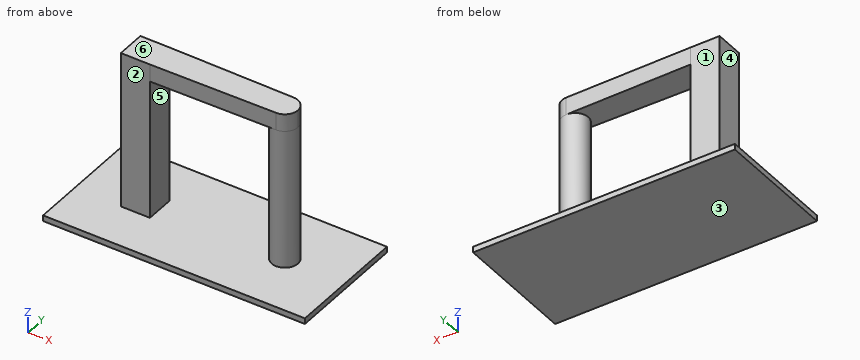
from build123d import *

# Parameters (mm, degrees)
F0_W     = 45
F0_H     = 21
F0_W_2   = 5
F0_H_2   = 5
F0_R     = 2.25
F1_DEPTH = 1
F2_DEPTH = 25
F3_W     = 5
F3_H     = 5
F4_DEPTH = 3


with BuildPart() as f1:
    # F0 (on Top) → F1 (new body)
    with BuildSketch(Plane.XY):
        Rectangle(F0_W, F0_H)
        with Locations((-12, 0)):
            Rectangle(F0_W_2, F0_H_2, mode=Mode.SUBTRACT)
        with Locations((12, 0)):
            Circle(F0_R, mode=Mode.SUBTRACT)
    extrude(amount=F1_DEPTH)

    # F0 (on Top) → F2 (join)
    with BuildSketch(Plane.XY):
        with Locations((-12, 0)):
            Rectangle(F0_W_2, F0_H_2)
        with Locations((12, 0)):
            Circle(F0_R)
    extrude(amount=F2_DEPTH)

    # F3 (on face) → F4 (join)
    with BuildSketch(Plane.XY.offset(25)):
        with BuildLine():
            Line((12.026145, 2.249848), (-9.5, 2.5))
            Line((-9.5, 2.5), (-9.5, -2.5))
            Line((-9.5, -2.5), (12.026145, -2.249848))
            ThreePointArc((12.026145, -2.249848), (9.75, 0), (12.026145, 2.249848))
        make_face()
        with Locations((-12, 0)):
            Rectangle(F3_W, F3_H)
        with BuildLine():
            ThreePointArc((14.25, 0), (13.600207, 1.58172), (12.026145, 2.249848))
            ThreePointArc((12.026145, 2.249848), (9.75, 0), (12.026145, -2.249848))
            ThreePointArc((12.026145, -2.249848), (13.600207, -1.58172), (14.25, 0))
        make_face()
    extrude(amount=F4_DEPTH)


solid = f1.part
The listing builds one solid part. Answer for the finished solid, in the listing's coordinates (mm). Face numbers are marked on the shaded views. A direction names the side the tool comes from. Give positions to 0.01 mm unless a question says otherwise; leave off trailing zeros. Write each loop counter-clockwise with the first axis right and the second up, starting at its lowest first coordinate (ties: lowest second). Pieces come first, ordered by that corner, then holes.
Item 1: Find the intervals of material crossed by line 1 along Z through (x, y) = (-5.5, 1.25); line 2 along Y through (x, z) = (-11, 16); line 3 along Z through (x, y) = (2, 6.5), in increasing order.
Item 2: Determine the mould class of the marked faces 4, 5 and 6 for opening direction Z: released by +Z, released by -Z, zero draft, split by the parting line, or undercut.
Item 3: Section C-C, the plane x = 3 is taken. Write down the section's boundary in (y, z), plus the area to 3 significant figures.
Item 4: Flat-ended cylindrical pins translate along their axes: P1, Ø2.5, axis at y = 1, z = 11, coming from the -X side; P2, Ø3, axis at x = 9, z = 13.5, coming from the +Y side; P3, Ø4, axis at y = 1, z = 9.5, coming from the +X side. Find the tip coordinate at first contact, or state that the pin passes through.
Item 5: Section B-B, the plane z = 9.25 is taken. Write down the section's boundary in (x, y).
Item 6: Which of the six approach directions +Z, -Z, +X, -X, +Y, -Y give full straight-line access (tool end or side, diameter ignored) to the marked faces 1, 2 and 3?
Item 7: Section D-D, the plane y = 5 is taken. Write down the section's boundary in (x, z).
Item 8: Section A-A, the plane x = -9 is taken. Write down the section's boundary in (y, z), plus the area to 3 significant figures.
Completed:
1. line 1: z = 0 to 1, 25 to 28
1. line 2: y = -2.5 to 2.5
1. line 3: z = 0 to 1
2. face 4: zero draft
2. face 5: undercut
2. face 6: released by +Z
3. outline: (-10.5, 0) - (10.5, 0) - (10.5, 1) - (-10.5, 1) - close; (-2.35, 25) - (2.35, 25) - (2.35, 28) - (-2.35, 28) - close
3. area: 35.1 mm2
4. P1: stops at x = -14.5
4. P2: stops at y = 1.68
4. P3: stops at x = 14.25
5. outline: (-14.5, -2.5) - (-9.5, -2.5) - (-9.5, 2.5) - (-14.5, 2.5) - close; circle Ø4.5 at (12, 0)
6. face 1: +Z, +X, -X, +Y
6. face 2: +Z, +X, -X, -Y
6. face 3: -Z, +X, -X, +Y, -Y
7. outline: (-22.5, 0) - (22.5, 0) - (22.5, 1) - (-22.5, 1) - close
8. outline: (-10.5, 0) - (10.5, 0) - (10.5, 1) - (-10.5, 1) - close; (-2.49, 25) - (2.49, 25) - (2.49, 28) - (-2.49, 28) - close
8. area: 36.0 mm2
